Part print with two shaded views. Sizes in mm from the minimum x, y, z corner. Round coordinates to 2 decimals unless told otherwise and drop trailing zeros. Answer as a JSON object with one key per item and string values.
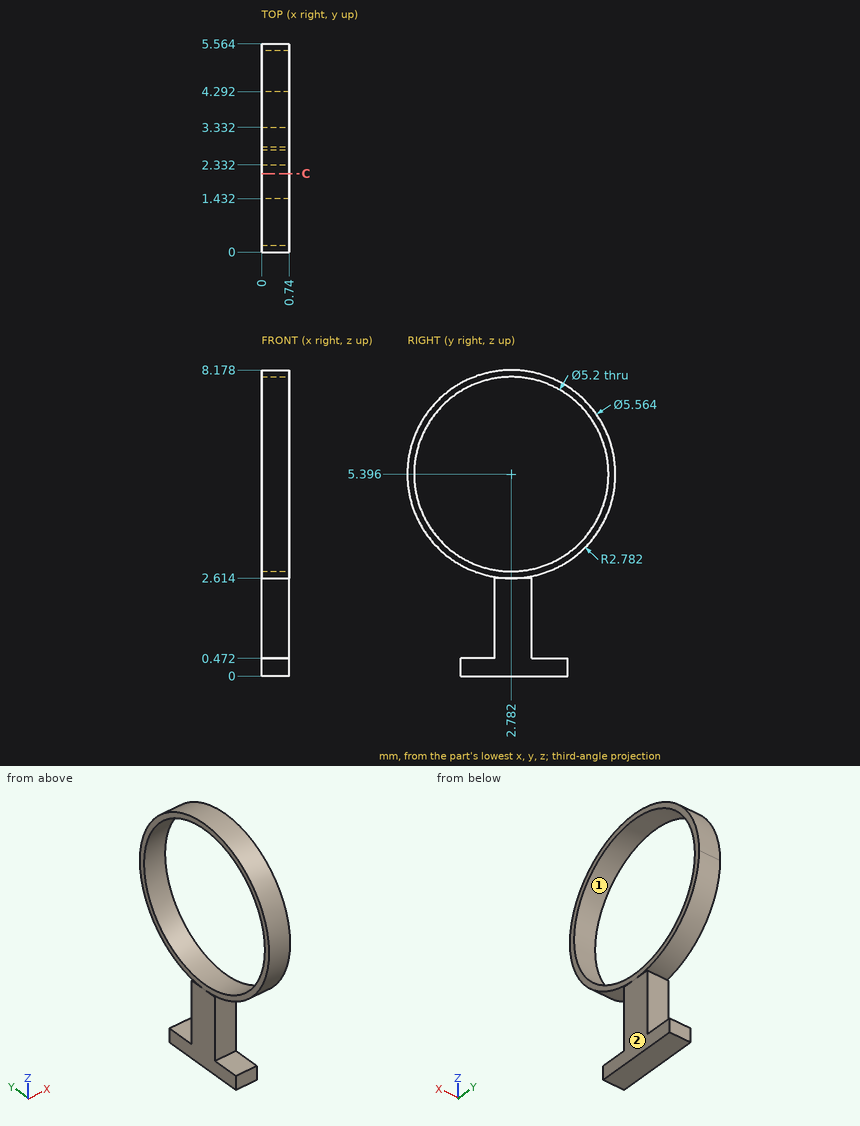
Item 1: Two-plate mould, pull along Y, no slides. Class the marked faces 1 and 2: released by +Y, released by -Y, zero draft, split by the parting line, or undercut.
Worked answers:
{"face 1": "undercut", "face 2": "zero draft"}
Item 2: Saw through at C-C on y = 2.1. State how many separate pieces and enclosed holes the cut face has.
Worked answers:
{"separate pieces": "3", "enclosed holes": "0"}
Item 3: Drop flat-ended pins along their axis: pin 1 Ø1.5 at (y, z) = (4.5, 2) entering from -X; pin 2 Ø1 at (y, z) = (2.5, 1.5) entering from -X. Give the stop position or say it passes through.
Worked answers:
{"pin 1": "passes through", "pin 2": "stops at x = 0"}
Item 4: Wall check: line 1 along Z through (x, y) = (0.3, 1.8) (1 decimal); line 2 along Y through (x, z) = (0.4, 6.5) (1 decimal); line 3 along Z through (x, y) = (0.5, 1.95). Give the ranges that are in metal, low to high. Write a range as [from, to].
Worked answers:
{"line 1": "z = [0, 0.5], [2.8, 3], [7.8, 8]", "line 2": "y = [0.2, 0.4], [5.1, 5.3]", "line 3": "z = [0, 0.47], [2.74, 2.93], [7.86, 8.05]"}
